The listing builds one solid part. Answer for the finished solid, in the listing's coordinates (mm). A direction names the side the tool comes from. Coordinates: 2 decimals unless noted, no trailing zeros. Order: outer loops, then holes, each group sorted by start corner. A loop starts at its lowest first (then second) coordinate and runs counter-clockwise, first axis right, second up.
```python
from build123d import *

# Parameters (mm, degrees)
SKETCH1_R           = 13
BOSS_EXTRUDE1_DEPTH = 2.5


with BuildPart() as part:
    # Sketch1 → Boss-Extrude1 (new, symmetric)
    with BuildSketch(Plane.XY):
        with BuildLine():
            Line((16, 23), (0, 23))
            Line((0, 23), (0, -23))
            Line((0, -23), (16, -23))
            Line((16, -23), (16, -18))
            Line((16, -18), (26, -18))
            Line((26, -18), (26, -23))
            Line((26, -23), (150, -23))
            ThreePointArc((150, -23), (173, 0), (150, 23))
            Line((150, 23), (26, 23))
            Line((26, 23), (26, 18))
            Line((26, 18), (16, 18))
            Line((16, 18), (16, 23))
        make_face()
        with Locations((150, 0)):
            Circle(SKETCH1_R, mode=Mode.SUBTRACT)
    extrude(amount=BOSS_EXTRUDE1_DEPTH, both=True)


solid = part.part
```
1) The mould has two halves that part along Y. Classify faces 4 (the cylindrical face through (172.994, -0.506, 0.035)), 5 (the cylindrical face through (162, -5, 0)), 6 (the flat face through (8, -23, 0)): released by +Y, released by -Y, zero draft, split by the parting line, or undercut.
2) For faces 1 (the flat face through (87, -23, 0)), 2 (the flat face through (16, -21, 0)), 3 (the flat face through (26, 21, 0)), determine the directions among +Z, -Z, +X, -X, +Y, -Y from which every point of the face is accessible in a straight line to the end or side of a thin tool.
3) This flat-tipped pin is pushed along its axis until it touches: P1, Ø2, axis at y = 8, z = -1, coming from the +X side. Where does it stop, or does it pass through?
4) A cutting plane is placed at A-A, the plane z = 0.3. Write down the section's boundary in (x, y), plus the area to 3 significant figures.
5) A cutting plane is placed at B-B, the plane y = 0. Write down the section's boundary in (x, z).
6) Straight lines are drawn through the part: probe 1 along Y at (x, z) = (150, 1.1); probe 2 along X at (y, z) = (-9, -1.5); probe 3 along X at (y, z) = (-19, 0.3). For each, find the intervals that lie inside material, in ascending order.
Working result:
1. face 4: split by the parting line
1. face 5: undercut
1. face 6: released by -Y
2. face 1: +Z, -Z, +X, -X, -Y
2. face 2: +Z, -Z, -Y
2. face 3: +Z, -Z, +Y
3. P1: stops at x = 171.91
4. outline: (0, -23) - (16, -23) - (16, -18) - (26, -18) - (26, -23) - (150, -23) arc R23 ccw to (150, 23) - (26, 23) - (26, 18) - (16, 18) - (16, 23) - (0, 23) - close; hole circle Ø26 at (150, 0)
4. area: 7,100 mm2
5. outline: (0, -2.5) - (137, -2.5) - (137, 2.5) - (0, 2.5) - close; (163, -2.5) - (173, -2.5) - (173, 2.5) - (163, 2.5) - close
6. probe 1: y = -23 to -13, 13 to 23
6. probe 2: x = 0 to 140.62, 159.38 to 171.17
6. probe 3: x = 0 to 16, 26 to 162.96
